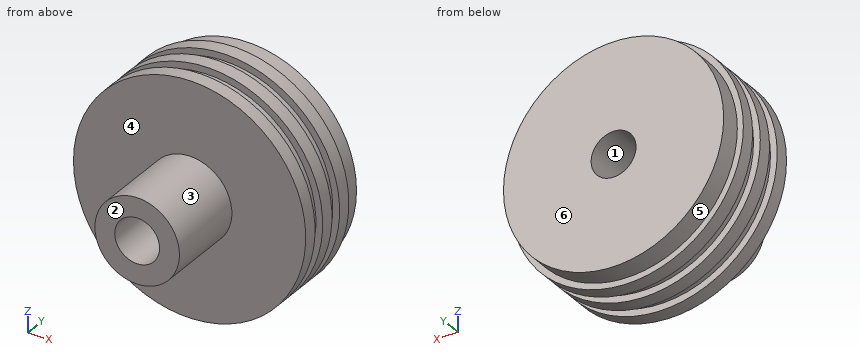
```python
from build123d import *

# Parameters (mm, degrees)
F_5_8_11_TAPPED_HOLE1_D = 13.49248


with BuildPart() as part:
    # Sketch8 → Revolve1 (revolve)
    with BuildSketch(Plane.XY):
        Polygon((0, 0), (0, 26.416), (-33.0835, 26.416), (-33.0835, 20.066), (-34.8996, 20.066), (-34.8996, 15.748), (-32.8676, 15.748), (-32.8676, 12.192), (-34.8996, 12.192), (-34.8996, 7.874), (-32.8676, 7.874), (-32.8676, 4.318), (-34.8996, 4.318), (-34.8996, 0), (-12.7, 0), (-12.7, -24.384), (0, -24.384), align=None)
    revolve(axis=Axis((0, 0, 0), (0, 1, 0)))

    # 5/8-11 Tapped Hole1 (through all)
    with Locations(Plane(origin=(0, 26.416, 0), x_dir=(1, 0, 0), z_dir=(0, 1, 0))):
        with Locations((0, 0)):
            Hole(F_5_8_11_TAPPED_HOLE1_D / 2)


solid = part.part
```
Can you work these out from the model? Positions are in its coordinate system, mm. Face numbers are marked on the shaded views. A direction names the side the tool comes from. Give positions to 0.01 mm unless a question says otherwise; leave off trailing zeros. Loops run counter-clockwise (first coordinate to the right, second up) from the corner with the lowest first, then second, coordinate; pieces in that order, holes last. Notation, with made-up numbers: M -5,-10.75 L 26,-10.75 A9 ccw 26,2.25 Z; hole C 77,15 d10. An arc over 180 degrees is marked long. One line per question, with ' | ' between items. Start each with the question number.
Q1. If we section it at D-D (x = 14): Please give me the cut outline in (y, z).
Q2. If I drill on line 1 (Y direction, x = 21, z = 27.5); line 2 (X direction, y = 5.5, z = 0.5); line 3 (Z direction, x = 0, y = -11), over which ranges is the centre line in solid material (lowest first)? Write a range as from..to.
Q3. If we mould it in two halves opening along Z, with no side actions, what happens to the marked faces 1, 2 and 3? For each: +Z half, -Z half, draft (parallel to the pull), parting line (faces both ways), or undercut.
Q4. For pin 1 Ø1.5 at (x, z) = (-13, -10) entering from -Y; pin 2 Ø4 at (y, z) = (20, 20.5) entering from -X; pin 3 Ø10 at (y, z) = (-0.5, -13.5) entering from -X, each with a flat end and sliding along its axis, tell me the tip position at first contact or that it passes through.
Q5. If we section it at C-C (y = -1): Please give me the cut outline in (x, z).
Q6. For the marked faces 4, 5 and 6, which set-ups out of +Z, -Z, +X, -X, +Y, -Y let a thin tool reach every point of the face, with its end or its side?
Computed:
1) outline: M 0,-31.97 L 4.32,-31.97 L 4.32,-29.74 L 7.87,-29.74 L 7.87,-31.97 L 12.19,-31.97 L 12.19,-29.74 L 15.75,-29.74 L 15.75,-31.97 L 20.07,-31.97 L 20.07,-29.98 L 26.42,-29.98 L 26.42,29.98 L 20.07,29.98 L 20.07,31.97 L 15.75,31.97 L 15.75,29.74 L 12.19,29.74 L 12.19,31.97 L 7.87,31.97 L 7.87,29.74 L 4.32,29.74 L 4.32,31.97 L 0,31.97 Z
2) line 1: y = 0..4.32, 7.87..12.19, 15.75..20.07 | line 2: x = -32.86..-6.73, 6.73..32.86 | line 3: z = -12.7..-6.75, 6.75..12.7
3) face 1: undercut | face 2: draft | face 3: parting line
4) pin 1: stops at y = 0 | pin 2: stops at x = -29.59 | pin 3: stops at x = -33.84
5) outline: C 0,0 d25.4; hole C 0,0 d13.49
6) face 4: -Y | face 5: +Y | face 6: +Z, -Z, +X, -X, +Y
